```python
from build123d import *

# Parameters (mm, degrees)
F0_W     = 30
F0_H     = 30
F0_R     = 1.25
F1_DEPTH = 5
F2_W     = 3
F2_H     = 30
F3_DEPTH = 5
F2_R     = 3.75
F2_R_2   = 1.25
F4_DEPTH = 3
F5_W     = 12
F5_H     = 3
F5_H_2   = 5
F6_DEPTH = 2
F7_W     = 12
F7_H     = 5
F7_H_2   = 3
F8_DEPTH = 2


# Not quite as in the source:
# - a feature names something its author has since deleted; it is built from what else it names


with BuildPart() as f1:
    # F0 (on Top) → F1 (new body)
    with BuildSketch(Plane.XY):
        with Locations((15, 15)):
            Rectangle(F0_W, F0_H)
        with Locations((15, 15)):
            Circle(F0_R, mode=Mode.SUBTRACT)
    extrude(amount=F1_DEPTH)

    # F2 (on face) → F3 (join)
    with BuildSketch(Plane.XY.offset(5)):
        with Locations((1.5, 15)):
            Rectangle(F2_W, F2_H)
        with Locations((28.5, 15)):
            Rectangle(F2_W, F2_H)
        Polygon((9, 3), (9, 0), (15, 0), (21, 0), (21, 3), (15, 3), align=None)
        Polygon((15, 30), (9, 30), (9, 27), (15, 27), (21, 27), (21, 30), align=None)
    extrude(amount=F3_DEPTH)

    # F2 (on face) → F4 (join)
    with BuildSketch(Plane.XY.offset(5)):
        with Locations((15, 15)):
            Circle(F2_R)
        with Locations((15, 15)):
            Circle(F2_R_2, mode=Mode.SUBTRACT)
    extrude(amount=F4_DEPTH)

    # F5 (on face) → F6 (join)
    with BuildSketch(Plane.XY.offset(10)):
        with Locations((15, 1.5)):
            Rectangle(F5_W, F5_H)
        with Locations((15, -2.5)):
            Rectangle(F5_W, F5_H_2)
    extrude(amount=F6_DEPTH)

    # F7 (on face) → F8 (join)
    with BuildSketch(Plane.XY.offset(10)):
        with Locations((15, 32.5)):
            Rectangle(F7_W, F7_H)
        with Locations((15, 28.5)):
            Rectangle(F7_W, F7_H_2)
    extrude(amount=F8_DEPTH)


solid = f1.part
```
Here's how the part is built. I have some questions about the finished solid (model axes, mm). A direction names the side the tool comes from. Coordinates: 2 decimals unless noted, no trailing zeros. Loops run counter-clockwise (first coordinate to the right, second up) from the corner with the lowest first, then second, coordinate; pieces in that order, holes last. Notation, with made-up numbers: (52, -38) - (98, -38) arc R11 cw to (98, -34) - close; hole circle Ø5 at (33.25, 82). An arc over 180 degrees is marked (long way). Answer as CSV lines item,"result".
Q1. If we section it at A-A, the plane z = 6.75: Write out the boundary of the cut face in (x, y).
Response:
outline,"(0, 0) - (3, 0) - (3, 30) - (0, 30) - close; (9, 0) - (21, 0) - (21, 3) - (9, 3) - close; (9, 27) - (21, 27) - (21, 30) - (9, 30) - close; circle Ø7.5 at (15, 15); (27, 0) - (30, 0) - (30, 30) - (27, 30) - close; hole circle Ø2.5 at (15, 15)"
Q2. For faces 1 (the face through (28, 15, 10)), 2 (the face through (14.19, 11.34, 6.48)), 3 (the face through (3, 15, 7)), 4 (the face through (15, 0, 4)), 5 (the face through (1, 15, 10)), which set-ups out of +Z, -Z, +X, -X, +Y, -Y let a thin tool reach every point of the face, with its end or its side?
Response:
face 1,"+Z, +X, +Y, -Y"
face 2,"+Z"
face 3,"+Z, +Y, -Y"
face 4,"-Z, +X, -X, -Y"
face 5,"+Z, -X, +Y, -Y"
Q3. If we section it at C-C, the plane y = 15: Write out the boundary of the cut face in (x, z).
Response:
outline,"(0, 0) - (13.75, 0) - (13.75, 8) - (11.25, 8) - (11.25, 5) - (3, 5) - (3, 10) - (0, 10) - close; (16.25, 0) - (30, 0) - (30, 10) - (27, 10) - (27, 5) - (18.75, 5) - (18.75, 8) - (16.25, 8) - close"
Q4. If we section it at D-D, the plane y = 28: Write out the boundary of the cut face in (x, z).
Response:
outline,"(0, 0) - (30, 0) - (30, 10) - (27, 10) - (27, 5) - (21, 5) - (21, 12) - (9, 12) - (9, 5) - (3, 5) - (3, 10) - (0, 10) - close"
Q5. For pin 1 (5 mm diameter, centred on x = 12, z = 6, fed in from -Y); pin 2 (0.9 mm diameter, centred on x = 1.5, y = 18.5, fed in from +Z); pin 3 (2 mm diameter, centred on x = 8, y = 21, fed in from +Z), each with a flat end and sliding along its axis, tell me the tip position at first contact or that it passes through.
Response:
pin 1,"y = 0"
pin 2,"z = 10"
pin 3,"z = 5"
Q6. If we section it at B-B, the plane x = 15: Write out the boundary of the cut face in (y, z).
Response:
outline,"(-5, 10) - (0, 10) - (0, 0) - (13.75, 0) - (13.75, 8) - (11.25, 8) - (11.25, 5) - (3, 5) - (3, 12) - (-5, 12) - close; (16.25, 0) - (30, 0) - (30, 10) - (35, 10) - (35, 12) - (27, 12) - (27, 5) - (18.75, 5) - (18.75, 8) - (16.25, 8) - close"
Q7. If I drill on L1, parallel to Y at x = 15, z = 5.25; L2, parallel to X at y = 13, z = 6.5; L3, parallel to Y at x = 11.75, z = 8.5, over which ranges is the centre line in solid material (lowest first)? Write a range as [from, to].
Response:
L1,"[0, 3], [11.25, 13.75], [16.25, 18.75], [27, 30]"
L2,"[0, 3], [11.83, 18.17], [27, 30]"
L3,"[0, 3], [27, 30]"
Q8. We'd pull the mould along Y, two halves only. Please class faces 6 (the face through (15, 33, 10)), 7 (the face through (14, 16, 8)), 8 (the face through (15, 27, 8)), 9 (the face through (15, -5, 11)): pulls with the +Y half, pulls with the -Y half, needs draft (parallel to the pull), parting line crosses it, or undercut.
Response:
face 6,"needs draft"
face 7,"undercut"
face 8,"undercut"
face 9,"pulls with the -Y half"
